```python
from build123d import *

# Parameters (mm, degrees)
F0_R     = 8.5
F1_DEPTH = 14
F2_R     = 11
F3_DEPTH = 7
F4_W     = 50
F4_H     = 60
F5_DEPTH = 5
F6_R     = 7
F7_R     = 17


with BuildPart() as f1:
    # F0 (on Right) → F1 (new body)
    with BuildSketch(Plane.YZ):
        with BuildLine():
            Line((21, -32), (15.821561, 2.382899))
            ThreePointArc((15.821561, 2.382899), (0, 16), (-15.821561, 2.382899))
            Line((-15.821561, 2.382899), (-21, -32))
            Line((-21, -32), (21, -32))
        make_face()
        Circle(F0_R, mode=Mode.SUBTRACT)
    extrude(amount=F1_DEPTH)

    # F2 (on face) → F3 (cut)
    with BuildSketch(Plane.YZ.offset(14)):
        Circle(F2_R)
    extrude(amount=-F3_DEPTH, mode=Mode.SUBTRACT)

    # F4 (on face) → F5 (join)
    with BuildSketch(Plane(origin=(0, 0, -32), x_dir=(1, 0, 0), z_dir=(0, 0, -1))):
        with Locations((-11, 0)):
            Rectangle(F4_W, F4_H)
    extrude(amount=-F5_DEPTH)

    # F6
    f6_edges = [f1.edges().sort_by_distance(p)[0] for p in [
        (7, -20.246946, -27),
        (0, 0, -27),
        (7, 20.246946, -27),
    ]]
    fillet(f6_edges, radius=F6_R)

    # F7
    f7_edges = [f1.edges().sort_by_distance(p)[0] for p in [
        (-36, -30, -29.5),
        (-36, 30, -29.5),
    ]]
    fillet(f7_edges, radius=F7_R)


solid = f1.part
```
Could you check a few things on this model? Use its own coordinates, in mm. A direction names the side the tool comes from. Round coordinates to 2 decimals unless told otherwise and drop trailing zeros. Loops run counter-clockwise (first coordinate to the right, second up) from the corner with the lowest first, then second, coordinate; pieces in that order, holes last. Notation, with made-up numbers: (36.25, 17.5) - (43.25, 17.5) arc R30 ccw to (43.25, 41.5) - close; hole circle Ø6 at (53.25, 18.5). An arc over 180 degrees is marked (long way). Answer in a Markdown table with one row per item. Add a question column.
(1) If we section it at B-B (z = 5.5): Please give me the cut outline in (x, y), plus the area to 3 significant figures.
(2) If we section it at D-D (x = -9.5): Please give me the cut outline in (y, z), plus the area to 3 significant figures.
(3) If we mould it in two halves opening along Y, with no side actions, what happens to faces 4 (the face through (5.69, -21.76, -25.35)), 5 (the face through (-31.15, 24.89, -29.46)), 6 (the face through (-36, 0, -30)), 7 (the face through (7, 3.2, -8.1))? For each: pulls with the +Y half, pulls with the -Y half, needs draft (parallel to the pull), parting line crosses it, or undercut.
(4) If we section it at C-C (z = -7): Please give me the cut outline in (x, y).
(5) For faces 1 (the face through (0, 0, -10)), 2 (the face through (10.55, -2.38, -10.74)), 3 (the face through (-11, 0, -32)), which set-ups out of +Z, -Z, +X, -X, +Y, -Y let a thin tool reach every point of the face, with its end or its side?
(6) If we section it at A-A (y = 0): Please give me the cut outline in (x, z), plus the area to 3 significant figures.
(7) I'm going to push flat-ended pins straight in: pin 1 (11 mm diameter, centred on y = 0.5, z = -6.5, fed in from -X); pin 2 (1.5 mm diameter, centred on y = -0.5, z = -8.5, fed in from +X); pin 3 (15 mm diameter, centred on x = -9, y = -10, fed in from +Z). Where does each tip first touch, or does it pass through?
(8) I need wall thicknesses on line 1 along Z through (x, y) = (2, 0); line 2 along Z through (x, y) = (9, 0); line 3 along X through (y, z) = (7.5, 8.5). Which ranges of each line are inside material? Lowest first, please.
Model answer:
| question | item | result |
|---|---|---|
| 1 | outline | (0, -15.02) - (14, -15.02) - (14, -9.53) - (7, -9.53) - (7, -6.48) - (0, -6.48) - close; (0, 6.48) - (7, 6.48) - (7, 9.53) - (14, 9.53) - (14, 15.02) - (0, 15.02) - close |
| 1 | area | 197 mm² |
| 2 | outline | (-30, -32) - (30, -32) - (30, -27) - (-30, -27) - close |
| 2 | area | 300 mm² |
| 3 | face 4 | pulls with the -Y half |
| 3 | face 5 | pulls with the +Y half |
| 3 | face 6 | needs draft |
| 3 | face 7 | undercut |
| 4 | outline | (0, -17.23) - (14, -17.23) - (14, -8.49) - (7, -8.49) - (7, -4.82) - (0, -4.82) - close; (0, 4.82) - (7, 4.82) - (7, 8.49) - (14, 8.49) - (14, 17.23) - (0, 17.23) - close |
| 5 | face 1 | +Z, -X, +Y, -Y |
| 5 | face 2 | +X |
| 5 | face 3 | -Z, +X, -X, +Y, -Y |
| 6 | outline | (-36, -32) - (14, -32) - (14, -11) - (7, -11) - (7, -8.5) - (0, -8.5) - (0, -20) arc R7 cw to (-7, -27) - (-36, -27) - close; (0, 8.5) - (7, 8.5) - (7, 11) - (14, 11) - (14, 16) - (0, 16) - close |
| 6 | area | 590 mm² |
| 7 | pin 1 | stops at x = 0 |
| 7 | pin 2 | stops at x = 7 |
| 7 | pin 3 | stops at z = -24.33 |
| 8 | line 1 | z = -32 to -8.5, 8.5 to 16 |
| 8 | line 2 | z = -32 to -11, 11 to 16 |
| 8 | line 3 | x = 0 to 14 |
